Part model, mm, in its own coordinate system. Face numbers are marked on the shaded views. A direction names the side the tool comes from. Give positions to 0.01 mm unless a question says otherwise; leave off trailing zeros. Order: outer loops, then holes, each group sorted by start corner. A loop starts at its lowest first (then second) coordinate and runs counter-clockwise, first axis right, second up. Notation, with made-up numbers: (63, -19.75) - (112, -19.75) arc R25 ccw to (112, 8.25) - close; hole circle Ø8 at (-34, 19). An arc over 180 degrees is marked (long way). Use a Markdown table: item, result. Add a question column.
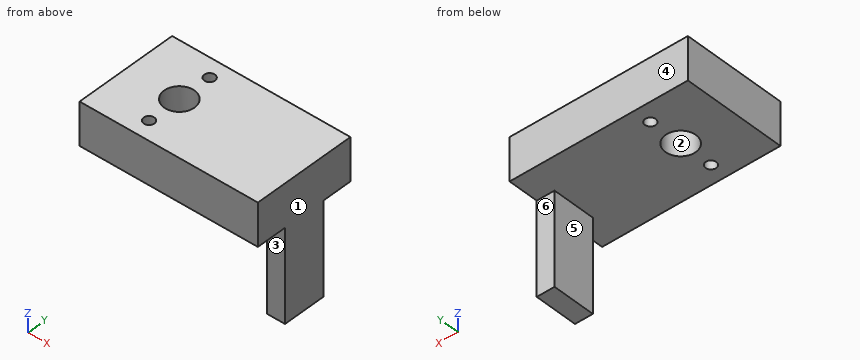
from build123d import *

# Parameters (mm, degrees)
SKETCH1_W           = 50
SKETCH1_H           = 29
BOSS_EXTRUDE1_DEPTH = 12
SKETCH2_R           = 4.25
CUT_EXTRUDE1_DEPTH  = 12
SKETCH6_R           = 1.5
CUT_EXTRUDE2_DEPTH  = 12
SKETCH3_W           = 5
SKETCH3_H           = 12
BOSS_EXTRUDE2_DEPTH = 26


with BuildPart() as part:
    # Sketch1 → Boss-Extrude1 (new body)
    with BuildSketch(Plane.XY):
        with Locations((-2.5, 0)):
            Rectangle(SKETCH1_W, SKETCH1_H)
    extrude(amount=BOSS_EXTRUDE1_DEPTH)

    # Sketch2 → Cut-Extrude1 (cut)
    with BuildSketch(Plane.XY.offset(12)):
        with Locations((-12.5, 0)):
            Circle(SKETCH2_R)
    extrude(amount=-CUT_EXTRUDE1_DEPTH, mode=Mode.SUBTRACT)

    # Sketch6 → Cut-Extrude2 (cut)
    with BuildSketch(Plane.XY.offset(12)):
        with Locations((-12.5, 9.5)):
            Circle(SKETCH6_R)
        with Locations((-12.5, -9.5)):
            Circle(SKETCH6_R)
    extrude(amount=-CUT_EXTRUDE2_DEPTH, mode=Mode.SUBTRACT)

    # Sketch3 → Boss-Extrude2 (add)
    with BuildSketch(Plane(origin=(0, 0, 0), x_dir=(-1, 0, 0), z_dir=(0, 0, -1))):
        with Locations((-20, 0)):
            Rectangle(SKETCH3_W, SKETCH3_H)
    extrude(amount=BOSS_EXTRUDE2_DEPTH)


solid = part.part
1. Drill centre lines: probe 1 along Y at (x, z) = (-12.5, 4.5); probe 2 along Y at (x, z) = (-12, 9); probe 3 along Z at (x, y) = (-17, -0.75). Where is each one in solid material? Low to high. Write a range as [from, to].
2. Cut at C-C (z = 2.5). Write the cut outline in (x, y), plus the area to 3 significant figures.
3. Mould opens along X. For the marked faces 1, 2 and 3 say: released by +X, released by -X, zero draft, split by the parting line, or undercut.
4. Cut at A-A (x = -12.5). Write the cut outline in (y, z), plus the area to 3 significant figures.
5. Tool access for the marked faces 4, 5 and 6: list every direction of +Z, -Z, +X, -X, +Y, -Y with a clear straight run to the whole face (end or side of a thin tool).
6. Cut at B-B (y = 9.5). Write the cut outline in (x, z).
7. Cut at D-D (y = 0). Write the cut outline in (x, z).
8. Pin check, flat tips, straight feed: P1, Ø3, axis at x = -16.5, y = 7, coming from the -Z side; P2, Ø5.5, axis at x = 21, z = -16, coming from the +Y side; P3, Ø3.5, axis at y = -2, z = -11.5, coming from the -X side; P4, Ø10, axis at y = -11, z = -3.5, coming from the -X side. Stop position of each tip, or through.
Responses:
| question | item | result |
|---|---|---|
| 1 | probe 1 | y = [-14.5, -11], [-8, -4.25], [4.25, 8], [11, 14.5] |
| 1 | probe 2 | y = [-14.5, -10.91], [-8.09, -4.22], [4.22, 8.09], [10.91, 14.5] |
| 1 | probe 3 | z = [0, 12] |
| 2 | outline | (-27.5, -14.5) - (22.5, -14.5) - (22.5, 14.5) - (-27.5, 14.5) - close; hole circle Ø8.5 at (-12.5, 0); hole circle Ø3 at (-12.5, -9.5); hole circle Ø3 at (-12.5, 9.5) |
| 2 | area | 1,380 mm² |
| 3 | face 1 | released by +X |
| 3 | face 2 | undercut |
| 3 | face 3 | zero draft |
| 4 | outline | (-14.5, 0) - (-11, 0) - (-11, 12) - (-14.5, 12) - close; (-8, 0) - (-4.25, 0) - (-4.25, 12) - (-8, 12) - close; (4.25, 0) - (8, 0) - (8, 12) - (4.25, 12) - close; (11, 0) - (14.5, 0) - (14.5, 12) - (11, 12) - close |
| 4 | area | 174 mm² |
| 5 | face 4 | +Z, -Z, +X, -X, +Y |
| 5 | face 5 | -Z, -X, +Y, -Y |
| 5 | face 6 | -Z, +X, -X, +Y |
| 6 | outline | (-27.5, 0) - (-14, 0) - (-14, 12) - (-27.5, 12) - close; (-11, 0) - (22.5, 0) - (22.5, 12) - (-11, 12) - close |
| 7 | outline | (-27.5, 0) - (-16.75, 0) - (-16.75, 12) - (-27.5, 12) - close; (-8.25, 0) - (17.5, 0) - (17.5, -26) - (22.5, -26) - (22.5, 12) - (-8.25, 12) - close |
| 8 | P1 | stops at z = 0 |
| 8 | P2 | stops at y = 6 |
| 8 | P3 | stops at x = 17.5 |
| 8 | P4 | stops at x = -27.5 |
